```python
from build123d import *

# Parameters (mm, degrees)
ESQUISSE1_W      = 29.99994
ESQUISSE1_H      = 54.0004
ESQUISSE1_R      = 0.50038
ESQUISSE1_R_2    = 0.4826
ESQUISSE1_R_3    = 0.39878
ESQUISSE1_R_4    = 0.55118
ESQUISSE1_R_5    = 0.65024
ESQUISSE1_R_6    = 1.6002
ESQUISSE1_R_7    = 0.44958
ESQUISSE1_R_8    = 1.24968
ESQUISSE1_R_9    = 0.59944
ESQUISSE1_R_10   = 0.5
ESQUISSE1_R_11   = 0.4
EXTRUSION1_DEPTH = 1.6


with BuildPart() as part:
    # Esquisse1 → Extrusion1 (new body)
    with BuildSketch(Plane.XY):
        with Locations((14.99997, 27.0002)):
            Rectangle(ESQUISSE1_W, ESQUISSE1_H)
        with Locations((18.17624, 38.36416)):
            Circle(ESQUISSE1_R, mode=Mode.SUBTRACT)
        with Locations((18.17624, 34.55416)):
            Circle(ESQUISSE1_R, mode=Mode.SUBTRACT)
        with Locations((11.82624, 34.55416)):
            Circle(ESQUISSE1_R, mode=Mode.SUBTRACT)
        with Locations((11.82624, 38.36416)):
            Circle(ESQUISSE1_R, mode=Mode.SUBTRACT)
        with Locations((17.59966, 3.50012)):
            Circle(ESQUISSE1_R, mode=Mode.SUBTRACT)
        with Locations((12.40028, 3.50012)):
            Circle(ESQUISSE1_R, mode=Mode.SUBTRACT)
        with Locations((12.40028, 50.50028)):
            Circle(ESQUISSE1_R, mode=Mode.SUBTRACT)
        with Locations((17.59966, 50.50028)):
            Circle(ESQUISSE1_R, mode=Mode.SUBTRACT)
        with Locations((3.50012, 10.9601)):
            Circle(ESQUISSE1_R_2, mode=Mode.SUBTRACT)
        with Locations((3.50012, 16.0401)):
            Circle(ESQUISSE1_R_2, mode=Mode.SUBTRACT)
        with Locations((14.98854, 30.82036)):
            Circle(ESQUISSE1_R_3, mode=Mode.SUBTRACT)
        with Locations((14.98854, 33.36036)):
            Circle(ESQUISSE1_R_3, mode=Mode.SUBTRACT)
        with Locations((16.27124, 47.50054)):
            Circle(ESQUISSE1_R, mode=Mode.SUBTRACT)
        with Locations((13.73124, 47.50054)):
            Circle(ESQUISSE1_R, mode=Mode.SUBTRACT)
        with Locations((27.70124, 13.28928)):
            Circle(ESQUISSE1_R_3, mode=Mode.SUBTRACT)
        with Locations((27.70124, 10.74928)):
            Circle(ESQUISSE1_R_3, mode=Mode.SUBTRACT)
        with Locations((1.4986, 13.5001)):
            Circle(ESQUISSE1_R_4, mode=Mode.SUBTRACT)
        with Locations((7.8994, 13.5001)):
            Circle(ESQUISSE1_R_4, mode=Mode.SUBTRACT)
        with Locations((5.79882, 11.75004)):
            Circle(ESQUISSE1_R_4, mode=Mode.SUBTRACT)
        with Locations((5.79882, 15.25016)):
            Circle(ESQUISSE1_R_4, mode=Mode.SUBTRACT)
        with Locations((3.50012, 13.5001)):
            Circle(ESQUISSE1_R_5, mode=Mode.SUBTRACT)
        with Locations((1.4986, 27.0002)):
            Circle(ESQUISSE1_R_4, mode=Mode.SUBTRACT)
        with Locations((7.8994, 27.0002)):
            Circle(ESQUISSE1_R_4, mode=Mode.SUBTRACT)
        with Locations((5.79882, 25.25014)):
            Circle(ESQUISSE1_R_4, mode=Mode.SUBTRACT)
        with Locations((5.79882, 28.75026)):
            Circle(ESQUISSE1_R_4, mode=Mode.SUBTRACT)
        with Locations((3.50012, 27.0002)):
            Circle(ESQUISSE1_R_5, mode=Mode.SUBTRACT)
        with Locations((1.4986, 40.5003)):
            Circle(ESQUISSE1_R_4, mode=Mode.SUBTRACT)
        with Locations((7.8994, 40.5003)):
            Circle(ESQUISSE1_R_4, mode=Mode.SUBTRACT)
        with Locations((5.79882, 38.75024)):
            Circle(ESQUISSE1_R_4, mode=Mode.SUBTRACT)
        with Locations((5.79882, 42.25036)):
            Circle(ESQUISSE1_R_4, mode=Mode.SUBTRACT)
        with Locations((3.50012, 40.5003)):
            Circle(ESQUISSE1_R_5, mode=Mode.SUBTRACT)
        with Locations((15.00124, 36.45916)):
            Circle(ESQUISSE1_R_3, mode=Mode.SUBTRACT)
        with Locations((15.00124, 41.53916)):
            Circle(ESQUISSE1_R_3, mode=Mode.SUBTRACT)
        with Locations((4.0005, 49.9999)):
            Circle(ESQUISSE1_R_6, mode=Mode.SUBTRACT)
        with Locations((25.99944, 49.9999)):
            Circle(ESQUISSE1_R_6, mode=Mode.SUBTRACT)
        with Locations((4.0005, 4.0005)):
            Circle(ESQUISSE1_R_6, mode=Mode.SUBTRACT)
        with Locations((25.99944, 4.0005)):
            Circle(ESQUISSE1_R_6, mode=Mode.SUBTRACT)
        with Locations((18.80616, 11.38428)):
            Circle(ESQUISSE1_R_7, mode=Mode.SUBTRACT)
        with Locations((18.80616, 13.92428)):
            Circle(ESQUISSE1_R_7, mode=Mode.SUBTRACT)
        with Locations((18.80616, 16.46428)):
            Circle(ESQUISSE1_R_7, mode=Mode.SUBTRACT)
        with Locations((18.80616, 19.00428)):
            Circle(ESQUISSE1_R_7, mode=Mode.SUBTRACT)
        with Locations((11.18616, 19.00428)):
            Circle(ESQUISSE1_R_7, mode=Mode.SUBTRACT)
        with Locations((11.18616, 16.46428)):
            Circle(ESQUISSE1_R_7, mode=Mode.SUBTRACT)
        with Locations((11.18616, 13.92428)):
            Circle(ESQUISSE1_R_7, mode=Mode.SUBTRACT)
        with Locations((11.18616, 11.38428)):
            Circle(ESQUISSE1_R_7, mode=Mode.SUBTRACT)
        with Locations((2.46126, 33.74898)):
            Circle(ESQUISSE1_R_3, mode=Mode.SUBTRACT)
        with Locations((5.00126, 33.74898)):
            Circle(ESQUISSE1_R_3, mode=Mode.SUBTRACT)
        with Locations((7.54126, 33.74898)):
            Circle(ESQUISSE1_R_3, mode=Mode.SUBTRACT)
        with Locations((2.46126, 20.24888)):
            Circle(ESQUISSE1_R_3, mode=Mode.SUBTRACT)
        with Locations((5.00126, 20.24888)):
            Circle(ESQUISSE1_R_3, mode=Mode.SUBTRACT)
        with Locations((7.54126, 20.24888)):
            Circle(ESQUISSE1_R_3, mode=Mode.SUBTRACT)
        with Locations((5.28066, 45.01134)):
            Circle(ESQUISSE1_R_3, mode=Mode.SUBTRACT)
        with Locations((2.74066, 45.01134)):
            Circle(ESQUISSE1_R_3, mode=Mode.SUBTRACT)
        with Locations((14.98854, 28.28036)):
            Circle(ESQUISSE1_R_3, mode=Mode.SUBTRACT)
        with Locations((14.98854, 25.74036)):
            Circle(ESQUISSE1_R_3, mode=Mode.SUBTRACT)
        with Locations((16.2814, 23.51024)):
            Circle(ESQUISSE1_R_3, mode=Mode.SUBTRACT)
        with Locations((13.7414, 23.51024)):
            Circle(ESQUISSE1_R_3, mode=Mode.SUBTRACT)
        with Locations((13.71854, 44.28744)):
            Circle(ESQUISSE1_R_3, mode=Mode.SUBTRACT)
        with Locations((16.25854, 44.28744)):
            Circle(ESQUISSE1_R_3, mode=Mode.SUBTRACT)
        with Locations((21.49856, 44.63542)):
            Circle(ESQUISSE1_R_4, mode=Mode.SUBTRACT)
        with Locations((21.49856, 39.55288)):
            Circle(ESQUISSE1_R_4, mode=Mode.SUBTRACT)
        with Locations((21.49856, 34.47288)):
            Circle(ESQUISSE1_R_4, mode=Mode.SUBTRACT)
        with Locations((25.69718, 42.84218)):
            Circle(ESQUISSE1_R_8, mode=Mode.SUBTRACT)
        with Locations((25.69718, 36.34232)):
            Circle(ESQUISSE1_R_8, mode=Mode.SUBTRACT)
        with Locations((23.50008, 29.5402)):
            Circle(ESQUISSE1_R, mode=Mode.SUBTRACT)
        with Locations((23.50008, 27.0002)):
            Circle(ESQUISSE1_R, mode=Mode.SUBTRACT)
        with Locations((23.50008, 24.4602)):
            Circle(ESQUISSE1_R, mode=Mode.SUBTRACT)
        with Locations((20.50034, 3.50012)):
            Circle(ESQUISSE1_R_3, mode=Mode.SUBTRACT)
        with Locations((9.4996, 3.50012)):
            Circle(ESQUISSE1_R_3, mode=Mode.SUBTRACT)
        with Locations((8.38454, 48.90262)):
            Circle(ESQUISSE1_R_3, mode=Mode.SUBTRACT)
        with Locations((8.38454, 37.90188)):
            Circle(ESQUISSE1_R_3, mode=Mode.SUBTRACT)
        with Locations((21.62048, 9.99998)):
            Circle(ESQUISSE1_R_3, mode=Mode.SUBTRACT)
        with Locations((21.62048, 21.00072)):
            Circle(ESQUISSE1_R_3, mode=Mode.SUBTRACT)
        with Locations((24.54402, 9.99998)):
            Circle(ESQUISSE1_R_3, mode=Mode.SUBTRACT)
        with Locations((24.54402, 21.00072)):
            Circle(ESQUISSE1_R_3, mode=Mode.SUBTRACT)
        with Locations((27.70124, 15.82928)):
            Circle(ESQUISSE1_R_3, mode=Mode.SUBTRACT)
        with Locations((27.70124, 37.1602)):
            Circle(ESQUISSE1_R_3, mode=Mode.SUBTRACT)
        with Locations((27.70124, 18.36928)):
            Circle(ESQUISSE1_R_3, mode=Mode.SUBTRACT)
        with Locations((27.70124, 35.0012)):
            Circle(ESQUISSE1_R_3, mode=Mode.SUBTRACT)
        with Locations((27.31008, 27.0002)):
            Circle(ESQUISSE1_R_9, mode=Mode.SUBTRACT)
        with Locations((27.31008, 29.5402)):
            Circle(ESQUISSE1_R_9, mode=Mode.SUBTRACT)
        with Locations((27.31008, 32.0802)):
            Circle(ESQUISSE1_R_9, mode=Mode.SUBTRACT)
        with Locations((27.31008, 24.4602)):
            Circle(ESQUISSE1_R_9, mode=Mode.SUBTRACT)
        with Locations((27.31008, 21.9202)):
            Circle(ESQUISSE1_R_9, mode=Mode.SUBTRACT)
        with Locations((19.19986, 27.0002)):
            Circle(ESQUISSE1_R_9, mode=Mode.SUBTRACT)
        with Locations((19.19986, 24.50084)):
            Circle(ESQUISSE1_R_3, mode=Mode.SUBTRACT)
        with Locations((11.00328, 32.07004)):
            Circle(ESQUISSE1_R_3, mode=Mode.SUBTRACT)
        with Locations((11.00328, 29.53004)):
            Circle(ESQUISSE1_R_3, mode=Mode.SUBTRACT)
        with Locations((11.00328, 26.99004)):
            Circle(ESQUISSE1_R_3, mode=Mode.SUBTRACT)
        with Locations((11.00328, 24.45004)):
            Circle(ESQUISSE1_R_3, mode=Mode.SUBTRACT)
        with Locations((11.00328, 21.91004)):
            Circle(ESQUISSE1_R_3, mode=Mode.SUBTRACT)
        with Locations((15.00124, 38.99916)):
            Circle(ESQUISSE1_R_3, mode=Mode.SUBTRACT)
        with Locations((14.99997, 7.50012)):
            Circle(ESQUISSE1_R_10, mode=Mode.SUBTRACT)
        with Locations((18.80997, 7.50012)):
            Circle(ESQUISSE1_R_11, mode=Mode.SUBTRACT)
    extrude(amount=EXTRUSION1_DEPTH)


solid = part.part
```
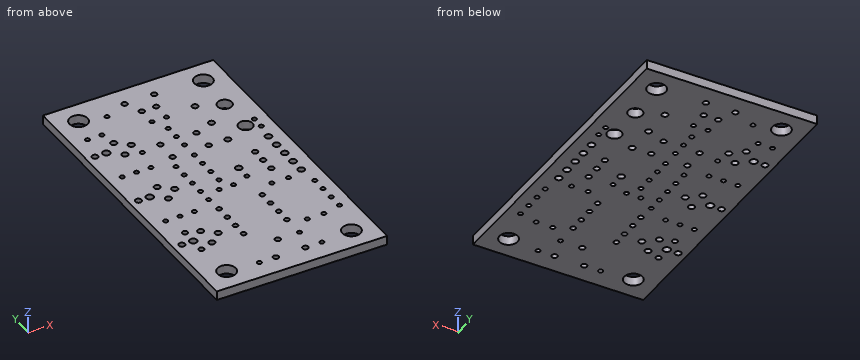
Check sheet for the modelled part. Datum: model origin and axes. Units: mm. Round coordinates to 2 decimals unless told otherwise and drop trailing zeros. Answer as a JSON object with one key per item and string values. Group by question number.
Q1. Gauge pin test, flat end, axial feed: P1, Ø1.4, axis at x = 27.31, y = 24.46, coming from the -Z side. Record the tip position at first contact, or that the pin passes through.
Q2. Sectioned sample at A-A, the plane z = 1.05. Count the separate pieces of the cut face and the enclosed holes in it, plus the area to 3 significant figures.
Q3. Scan lines: line 1 along X through (y, z) = (29.5, 0.7); line 2 along Y through (x, z) = (23.5, 0.2); line 3 along X through (y, z) = (21, 0.3). Record each from-to range of solid material in increasing order. Write a range as [from, to].
Solution:
{
 "1": {"P1": "stops at z = 0"},
 "2": {"separate pieces": "1", "enclosed holes": "94", "area": "1,520 mm²"},
 "3": {"line 1": "x = [0, 10.61], [11.4, 23], [24, 26.71], [27.91, 30]", "line 2": "y = [0, 23.96], [24.96, 26.5], [27.5, 29.04], [30.04, 54]", "line 3": "x = [0, 21.22], [22.02, 24.15], [24.94, 30]"}
}
